from build123d import *

# Parameters (mm, degrees)
F0_W      = 6
F0_H      = 6
F0_R      = 2.05
F1_DEPTH  = 15
F3_W      = 6
F3_H      = 6
F4_DEPTH  = 3
F8_R      = 2.65
F8_R_2    = 1.5
F10_DEPTH = 10
F11_DEPTH = 8.02


with BuildPart() as f1:
    # F0 (on Top) → F1 (new body)
    with BuildSketch(Plane.XY):
        Rectangle(F0_W, F0_H)
        Circle(F0_R, mode=Mode.SUBTRACT)
    extrude(amount=F1_DEPTH)

    # F3 (on offset) → F4 (join)
    with BuildSketch(Plane.XY.offset(15)):
        Rectangle(F3_W, F3_H)
    extrude(amount=F4_DEPTH)

    # F8 (on offset) → F9 (join, up to the next surface of F1)
    with BuildSketch(Plane(origin=(11.349514303, 0, 6.552645138), x_dir=(0, -1, 0), z_dir=(-0.8660254038, 0, -0.5))):
        with Locations((0, 11.3801583648)):
            Circle(F8_R)
        with Locations((0, 11.3801583648)):
            Circle(F8_R_2, mode=Mode.SUBTRACT)
    extrude(until=Until.NEXT)

    # F8 (on offset) → F10 (join)
    with BuildSketch(Plane(origin=(11.349514303, 0, 6.552645138), x_dir=(0, -1, 0), z_dir=(-0.8660254038, 0, -0.5))):
        with Locations((0, 11.3801583648)):
            Circle(F8_R)
        with Locations((0, 11.3801583648)):
            Circle(F8_R_2, mode=Mode.SUBTRACT)
    extrude(amount=-F10_DEPTH)

    # F8 (on offset) → F11 (cut)
    with BuildSketch(Plane(origin=(11.349514303, 0, 6.552645138), x_dir=(0, -1, 0), z_dir=(-0.8660254038, 0, -0.5))):
        with Locations((0, 11.3801583648)):
            Circle(F8_R_2)
    extrude(amount=F11_DEPTH, mode=Mode.SUBTRACT)


solid = f1.part
Input: part model. Units: mm. Frame: model coordinates. A direction names the side the tool comes from. Round coordinates to 2 decimals unless told otherwise and drop trailing zeros. Order: outer loops, then holes, each group sorted by start corner. A loop starts at its lowest first (then second) coordinate and runs counter-clockwise, first axis right, second up. Notation, with made-up numbers: (-25.75, 32) - (26.25, 32) arc R14 ccw to (26.25, 58) - close; hole circle Ø6 at (64.25, -34.5). An arc over 180 degrees is marked (long way). Answer as a JSON object with one key per item and string values. Group by question number.
(1) Reachability of faces 5 (the face through (-2.05, 0.09, 7.4)), 6 (the face through (0, 0, 18)), 7 (the face through (0, -3, 9)) from +Z, -Z, +X, -X, +Y, -Y: full face, straight path, thin tool, end or side. Return the list, or none.
(2) Draft query along X for faces 1 (the face through (0, 3, 9)), 2 (the face through (15.184, 0.037, 19.91)), 3 (the face through (-3, 0, 9)), 4 (the face through (0, 0, 15)). Return one class per face: released by +X, released by -X, zero draft, split by the parting line, or undercut.
(3) Pin query (flat end, axial travel): P1, Ø1, axis at y = 1.5, z = 20, coming from the -X side; P2, Ø2, axis at x = 13.5, y = -2.5, coming from the +Z side; P3, Ø1.8, axis at y = -1, z = 5, coming from the +X side. Return the tip coordinate at first contact, or that it passes through.
(4) Cut plane A-A (z = 4). Return loops of the section in (x, y), then the cut area to 3 significant figures.
(5) Cut plane B-B (y = 1). Return loops of the section in (x, z).
(6) Cut plane C-C (y = 2.4). Return loops of the section in (x, z).
(7) Material intervals for probe 1 along Y at (x, z) = (0, 10); probe 2 along Z at (x, y) = (7, 0.25), sorted ascending. Write a range as from..to.
Here are the results:
{
 "1": {"face 5": "-Z", "face 6": "+Z, -X, +Y, -Y", "face 7": "+Z, -Z, +X, -X, -Y"},
 "2": {"face 1": "zero draft", "face 2": "released by +X", "face 3": "released by -X", "face 4": "undercut"},
 "3": {"P1": "stops at x = 6.46", "P2": "stops at z = 23.28", "P3": "stops at x = 3"},
 "4": {"outline": "(-3, -3) - (3, -3) - (3, 3) - (-3, 3) - close; hole circle Ø4.1 at (0, 0)", "area": "22.8 mm^2"},
 "5": {"outline": "(-3, 0) - (-1.79, 0) - (-1.79, 13.27) - (-1.85, 13.37) - (-1.79, 13.4) - (-1.79, 15) - (0.98, 15) - (13.76, 22.38) - (13.09, 23.53) - (3, 17.71) - (3, 18) - (-3, 18) - close; (1.79, 0) - (3, 0) - (3, 12.04) - (15.55, 19.28) - (14.88, 20.44) - (1.79, 12.88) - close"},
 "6": {"outline": "(-3, 0) - (3, 0) - (3, 13.58) - (14.88, 20.44) - (13.76, 22.38) - (3, 16.17) - (3, 18) - (-3, 18) - close"},
 "7": {"probe 1": "y = -3..-2.05, 2.05..3", "probe 2": "z = 14.14..15.47, 18.89..20.23"}
}
